```python
from build123d import *

# Parameters (mm, degrees)
F3_DEPTH = 15
F5_DEPTH = 10


with BuildPart() as f1:
    # F0 (on Top) → F1 (revolve)
    with BuildSketch(Plane.XY):
        Polygon((-100, 0), (0, 0), (0, 120), (-34.996529, 120.492912), align=None)
    revolve(axis=Axis((0, 60, 0), (0, 1, 0)))

    # F2 (on Top) → F3 (join, symmetric)
    with BuildSketch(Plane.XY):
        with BuildLine():
            ThreePointArc((5, 150), (-3.535534, 153.535534), (0, 145))
            ThreePointArc((0, 145), (3.535534, 146.464466), (5, 150))
        make_face()
        with BuildLine():
            Line((-10, 120), (0, 120))
            Line((0, 120), (10, 120))
            Line((10, 120), (10, 150))
            ThreePointArc((10, 150), (0, 160), (-10, 150))
            Line((-10, 150), (-10, 120))
        make_face()
        with BuildLine():
            ThreePointArc((5, 150), (3.535534, 146.464466), (0, 145))
            ThreePointArc((0, 145), (-3.535534, 153.535534), (5, 150))
        make_face(mode=Mode.SUBTRACT)
    extrude(amount=F3_DEPTH, both=True)

    # F4 (on Top) → F5 (cut, symmetric)
    with BuildSketch(Plane.XY):
        with BuildLine():
            ThreePointArc((5, 150), (-3.535534, 153.535534), (0, 145))
            ThreePointArc((0, 145), (3.535534, 146.464466), (5, 150))
        make_face()
        with BuildLine():
            Line((-10, 120), (0, 120))
            Line((0, 120), (10, 120))
            Line((10, 120), (10, 150))
            ThreePointArc((10, 150), (0, 160), (-10, 150))
            Line((-10, 150), (-10, 120))
        make_face()
        with BuildLine():
            ThreePointArc((5, 150), (3.535534, 146.464466), (0, 145))
            ThreePointArc((0, 145), (-3.535534, 153.535534), (5, 150))
        make_face(mode=Mode.SUBTRACT)
    extrude(amount=F5_DEPTH, both=True, mode=Mode.SUBTRACT)


solid = f1.part
```
CAD build for the part. Positions are in the model's coordinates, mm. Give positions to 0.01 mm unless a question says otherwise; leave off trailing zeros. Order: outer loops, then holes, each group sorted by start corner. A loop starts at its lowest first (then second) coordinate and runs counter-clockwise, first axis right, second up.
(1) Saw through at B-B, the plane y = 111.5. Give the cut face in (x, z), then the cut area to 3 significant figures.
(2) Drill centre lines: L1, parallel to X at y = 150, z = 12.2; L2, parallel to Z at x = -13.5, y = 10.5; L3, parallel to Y at x = 7, z = -68.5. Where is each one in solid material? Low to high.
(3) Mould opens along Z. For faces 1 (the flat face through (0, 120, 0)), 2 (the conical face through (6.97, 86.18, 53.05)), 3 (the cylindrical face through (0, 160, -12)) say: released by +Z, released by -Z, zero draft, split by the parting line, or undercut.
(4) Flat gauge pins, fed straight in: pin 1 (2.5 mm diameter, centred on y = 138.5, z = -12, fed in from -X); pin 2 (1.5 mm diameter, centred on y = 73, z = -5.5, fed in from +X); pin 3 (22 mm diameter, centred on x = -1, y = 138, fed in from +Z). Where does each tip first touch, or does it go through?
(5) Saw through at C-C, the plane y = 49. Give the cut face in (x, z).
(6) Saw through at A-A, the plane z = 0. Give the cut face in (x, y), then the cut area to 3 significant figures.
Results found:
1. outline: circle Ø79.7 at (0, 0)
1. area: 4,990 mm2
2. L1: x = -10 to -5, 5 to 10
2. L2: z = -93.36 to 93.36
2. L3: y = 0 to 57.73
3. face 1: undercut
3. face 2: split by the parting line
3. face 3: zero draft
4. pin 1: stops at x = -10
4. pin 2: stops at x = 60.78
4. pin 3: stops at z = 15
5. outline: circle Ø147.13 at (0, 0)
6. outline: (-100, 0) - (100, 0) - (35, 120.49) - (10, 120.14) - (10, 120) - (-10, 120) - (-10, 120.14) - (-35, 120.49) - close
6. area: 16,200 mm2
